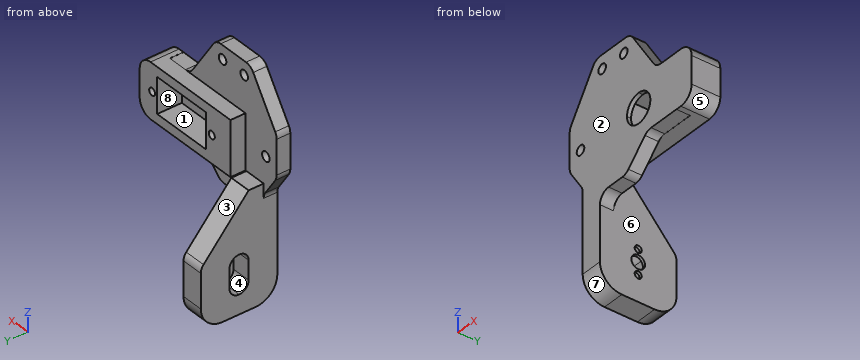
from build123d import *

# Parameters (mm, degrees)
BOSS_EXTRUDE1_DEPTH = 5
SKETCH2_R           = 1.75
SKETCH2_W           = 10.8
SKETCH2_H           = 10.8
CUT_EXTRUDE1_DEPTH  = 54.252895531
FILLET1_R           = 5.4
FILLET2_R           = 5.4
FILLET3_RADIUS      = 10
FILLET3_LENGTH      = 5
SKETCH6_W           = 35
SKETCH6_H           = 20.042215846
SKETCH6_W_2         = 23
SKETCH6_H_2         = 13
BOSS_EXTRUDE3_DEPTH = 5.5
SKETCH7_W           = 23
SKETCH7_H           = 13
CUT_EXTRUDE3_DEPTH  = 3.5
CUT_EXTRUDE4_DEPTH  = 54.302165833
SKETCH9_W           = 8
SKETCH9_H           = 28
BOSS_EXTRUDE4_DEPTH = 32
SKETCH11_R          = 2.5
SKETCH11_R_2        = 1.3
CUT_EXTRUDE5_DEPTH  = 69.854164991
FILLET6_R           = 8
BOSS_EXTRUDE5_DEPTH = 8
SKETCH13_W          = 14
SKETCH13_H          = 7
CUT_EXTRUDE6_DEPTH  = 7
FILLET7_R           = 3.5
FILLET8_R           = 3.5
CUT_EXTRUDE7_DEPTH  = 74.28896148
FILLET9_R           = 4
SKETCH15_W          = 5.3
SKETCH15_H          = 13
SKETCH15_R          = 1.4
BOSS_EXTRUDE6_DEPTH = 9
SKETCH16_W          = 7
SKETCH16_H          = 20.042215846
BOSS_EXTRUDE7_DEPTH = 10.5
SKETCH17_R          = 1.35
CUT_EXTRUDE8_DEPTH  = 9
FILLET10_R          = 5
SKETCH18_W          = 4.9
SKETCH18_H          = 13
CUT_EXTRUDE9_DEPTH  = 9


# Some blends are built 0.0001 mm under size
with BuildPart() as part:
    # Sketch1 → Boss-Extrude1 (new body)
    with BuildSketch(Plane(origin=(0, 0, 0), x_dir=(1, 0, 0), z_dir=(0, 1, 0))):
        Polygon((45, -10), (45, 10), (21, 10), (11.001510114, 19.998489886), (-4.998489886, 19.998489886), (-14.999716743, 4.996611292), (-14.999716743, -10.003388708), (-2.979747437, -28.033388708), (13.020252563, -28.033388708), (25.042481003, -10), align=None)
    extrude(amount=BOSS_EXTRUDE1_DEPTH)

    # Sketch2 → Cut-Extrude1 (cut, through all)
    with BuildSketch(Plane(origin=(0, 5, 0), x_dir=(1, 0, 0), z_dir=(0, 1, 0))):
        with Locations(Location((-9.999716743, 0, 0), (0, 0, 270))):
            Circle(SKETCH2_R)
        with Locations(Location((0.02138213, -23.033388708, 0), (0, 0, 270))):
            Circle(SKETCH2_R)
        with Locations(Location((10.02138213, -23.033388708, 0), (0, 0, 270))):
            Circle(SKETCH2_R)
        with Locations((16.9, 0)):
            Rectangle(SKETCH2_W, SKETCH2_H)
    extrude(amount=-CUT_EXTRUDE1_DEPTH, mode=Mode.SUBTRACT)

    # Fillet1
    fillet1_edges = [part.edges().sort_by_distance(p)[0] for p in [
        (11.5, 2.5, 5.4),
        (11.5, 2.5, -5.4),
    ]]
    fillet(fillet1_edges, radius=FILLET1_R - 0.0001)  # a hair under: the kernel refuses the full size

    # Fillet2
    # the kernel refuses this fillet: 5.4 mm, written as the material it adds along each edge
    with BuildSketch(Plane(origin=(22.3, 5, 5.4), x_dir=(-1, 0, 0), z_dir=(0, -1, 0)), Plane(origin=(22.3, 5, -5.4), x_dir=(0, 0, 1), z_dir=(0, -1, 0))) as fillet2_piece_1:
        with BuildLine():
            CenterArc((FILLET2_R, FILLET2_R), FILLET2_R, 180, 90)
            Line((0, FILLET2_R), (0, 0))
            Line((0, 0), (FILLET2_R, 0))
        make_face()
    extrude(amount=5)
    # the kernel refuses this fillet: 5.4 mm, written as the material it takes off along each edge

    # Fillet3: full round fillet: the end face becomes a half cylinder, R = half its width
    fillet3_face = Plane((45, 2.5, 0), x_dir=(0, 1, 0), z_dir=(1, 0, 0))  # on the end face: x along it, z out of the body
    fillet3_slab = fillet3_face.offset(-FILLET3_RADIUS / 2) * Box(FILLET3_LENGTH, 2 * FILLET3_RADIUS, FILLET3_RADIUS, mode=Mode.PRIVATE)  # the body's end, R deep
    fillet3_round = Plane((35, 2.5, 0), x_dir=(1, 0, 0), z_dir=(0, 1, 0)) * Cylinder(FILLET3_RADIUS, FILLET3_LENGTH, mode=Mode.PRIVATE)  # its axis R under the face
    add(fillet3_slab - fillet3_round, mode=Mode.SUBTRACT)

    # Sketch6 → Boss-Extrude3 (add)
    with BuildSketch(Plane(origin=(0, 5, 0), x_dir=(1, 0, 0), z_dir=(0, 1, 0))):
        with Locations((16.9, 0)):
            Rectangle(SKETCH6_W, SKETCH6_H)
        with Locations((16.9, 0)):
            Rectangle(SKETCH6_W_2, SKETCH6_H_2, mode=Mode.SUBTRACT)
    extrude(amount=BOSS_EXTRUDE3_DEPTH)

    # Sketch7 → Cut-Extrude3 (cut)
    with BuildSketch(Plane(origin=(0, 5, 0), x_dir=(1, 0, 0), z_dir=(0, 1, 0))):
        with Locations((16.9, 0)):
            Rectangle(SKETCH7_W, SKETCH7_H)
    extrude(amount=-CUT_EXTRUDE3_DEPTH, mode=Mode.SUBTRACT)

    # Sketch8 → Cut-Extrude4 (cut, through all)
    with BuildSketch(Plane(origin=(0, 5, 0), x_dir=(1, 0, 0), z_dir=(0, 1, 0))):
        with BuildLine():
            Line((34.4, 10), (34.4, -10))
            Line((34.4, -10), (35, -10))
            ThreePointArc((35, -10), (45, 0), (35, 10))
            Line((35, 10), (34.4, 10))
        make_face()
    extrude(amount=-CUT_EXTRUDE4_DEPTH, mode=Mode.SUBTRACT)

    # Sketch9 → Boss-Extrude4 (add)
    with BuildSketch(Plane(origin=(0, 0, -19.998489886), x_dir=(-1, 0, 0), z_dir=(0, 0, -1))):
        with Locations((4.998489886, 14)):
            Rectangle(SKETCH9_W, SKETCH9_H)
    extrude(amount=BOSS_EXTRUDE4_DEPTH)

    # Sketch11 → Cut-Extrude5 (cut, through all)
    with BuildSketch(Plane(origin=(-0.998489886, 0, 0), x_dir=(0, 0, -1), z_dir=(1, 0, 0))):
        with Locations((37.998489886, 14)):
            Circle(SKETCH11_R)
        with Locations((33.498489886, 14)):
            Circle(SKETCH11_R_2)
        with Locations((42.498489886, 14)):
            Circle(SKETCH11_R_2)
    extrude(amount=-CUT_EXTRUDE5_DEPTH, mode=Mode.SUBTRACT)

    # Fillet6
    fillet6_edges = [part.edges().sort_by_distance(p)[0] for p in [
        (-4.998489886, 0, -51.998489886),
        (-4.998489886, 28, -51.998489886),
    ]]
    fillet(fillet6_edges, radius=FILLET6_R)

    # Sketch12 → Boss-Extrude5 (add)
    with BuildSketch(Plane.ZY.offset(8.998489886)):
        Polygon((-10.021107923, 10.5), (-19.998489886, 28), (-19.998489886, 0), (-10, 0), align=None)
    extrude(amount=-BOSS_EXTRUDE5_DEPTH)

    # Sketch13 → Cut-Extrude6 (cut)
    with BuildSketch(Plane.ZY.offset(8.998489886)):
        with Locations((-37.998489886, 14)):
            Rectangle(SKETCH13_W, SKETCH13_H)
    extrude(amount=-CUT_EXTRUDE6_DEPTH, mode=Mode.SUBTRACT)

    # Fillet7
    fillet7_edges = [part.edges().sort_by_distance(p)[0] for p in [
        (-5.498489886, 10.5, -44.998489886),
        (-5.498489886, 17.5, -44.998489886),
    ]]
    fillet(fillet7_edges, radius=FILLET7_R - 0.0001)  # a hair under: the kernel refuses the full size

    # Fillet8
    fillet8_edges = [part.edges().sort_by_distance(p)[0] for p in [
        (-5.498489886, 17.5, -30.998489886),
        (-5.498489886, 10.5, -30.998489886),
    ]]
    fillet(fillet8_edges, radius=FILLET8_R - 0.0001)  # a hair under: the kernel refuses the full size

    # Sketch14 → Cut-Extrude7 (cut, through all)
    with BuildSketch(Plane.ZY.offset(8.998489886)):
        Polygon((-10.021107923, 10.5), (-29.998489886, 28), (-19.998489886, 28), align=None)
    extrude(amount=-CUT_EXTRUDE7_DEPTH, mode=Mode.SUBTRACT)

    # Fillet9
    # the kernel refuses this fillet: 4 mm, written as the material it adds along each edge
    with BuildSketch(Plane(origin=(-0.998489886, 5, -19.998489886), x_dir=(1, 0, 0), z_dir=(0, -1, 0))) as fillet9_piece_1:
        with BuildLine():
            CenterArc((FILLET9_R, -FILLET9_R), FILLET9_R, 90, 90)
            Line((0, -FILLET9_R), (0, 0))
            Line((0, 0), (FILLET9_R, 0))
        make_face()
    extrude(amount=5)
    with BuildSketch(Plane(origin=(25.042481003, 0, 10), x_dir=(-0.5546992156114033, 0, 0.8320509480795595), z_dir=(0, 1, 0))) as fillet9_piece_2:
        with BuildLine():
            CenterArc((FILLET9_R * 0.535184516545, FILLET9_R), FILLET9_R, 213.69, 56.31)
            Line((-FILLET9_R * 0.296866431535, FILLET9_R * 0.445300784389), (0, 0))
            Line((0, 0), (FILLET9_R * 0.535184516545, 0))
        make_face()
    extrude(amount=5)
    with BuildSketch(Plane(origin=(21, 0, -10), x_dir=(1, 0, 0), z_dir=(0, 1, 0))) as fillet9_piece_3:
        with BuildLine():
            CenterArc((FILLET9_R * 0.414213562373, FILLET9_R), FILLET9_R, 225, 45)
            Line((-FILLET9_R * 0.292893218813, FILLET9_R * 0.292893218813), (0, 0))
            Line((0, 0), (FILLET9_R * 0.414213562373, 0))
        make_face()
    extrude(amount=5)
    with BuildSketch(Plane(origin=(-8.998489886, 5, -13.998474565), x_dir=(0, 0, -1), z_dir=(0, -1, 0))) as fillet9_piece_4:
        with BuildLine():
            CenterArc((FILLET9_R * 0.302774994436, -FILLET9_R), FILLET9_R, 90, 33.69)
            Line((-FILLET9_R * 0.251924221175, -FILLET9_R * 0.16794905192), (0, 0))
            Line((0, 0), (FILLET9_R * 0.302774994436, 0))
        make_face()
    extrude(amount=5)
    # the kernel refuses this fillet: 4 mm, written as the material it takes off along each edge
    with BuildSketch(Plane(origin=(13.020252563, -5.351845165, 28.033388708), x_dir=(0.5546992156114035, 0, -0.8320509480795594), z_dir=(0, 1, 0)), Plane(origin=(-2.979747437, -5.351845165, 28.033388708), x_dir=(1, 0, 0), z_dir=(0, 1, 0))) as fillet9_2_piece_1:
        with BuildLine():
            CenterArc((FILLET9_R * 0.535184516545, FILLET9_R), FILLET9_R, 213.69, 56.31)
            Line((-FILLET9_R * 0.296866431535, FILLET9_R * 0.445300784389), (0, 0))
            Line((0, 0), (FILLET9_R * 0.535184516545, 0))
        make_face()
    extrude(amount=15.703690331, mode=Mode.SUBTRACT)
    with BuildSketch(Plane(origin=(-14.999716743, -3.027749944, 10.003388708), x_dir=(0.5546992156114036, 0, 0.8320509480795593), z_dir=(0, 1, 0)), Plane(origin=(-14.999716743, -3.027749944, -4.996611292), x_dir=(0, 0, 1), z_dir=(0, 1, 0))) as fillet9_2_piece_2:
        with BuildLine():
            CenterArc((FILLET9_R * 0.302774994436, FILLET9_R), FILLET9_R, 236.31, 33.69)
            Line((-FILLET9_R * 0.251924221175, FILLET9_R * 0.16794905192), (0, 0))
            Line((0, 0), (FILLET9_R * 0.302774994436, 0))
        make_face()
    extrude(amount=11.055499889, mode=Mode.SUBTRACT)
    with BuildSketch(Plane(origin=(11.001510114, -4.142135624, -19.998489886), x_dir=(-1, 0, 0), z_dir=(0, 1, 0))) as fillet9_2_piece_3:
        with BuildLine():
            CenterArc((FILLET9_R * 0.414213562373, FILLET9_R), FILLET9_R, 225, 45)
            Line((-FILLET9_R * 0.292893218813, FILLET9_R * 0.292893218813), (0, 0))
            Line((0, 0), (FILLET9_R * 0.414213562373, 0))
        make_face()
    extrude(amount=13.284271247, mode=Mode.SUBTRACT)
    with BuildSketch(Plane(origin=(-12.759041279, 28, -29.998489886), x_dir=(0, -0.658926553885557, 0.7522072829908683), z_dir=(1, 0, 0))) as fillet9_2_piece_4:
        with BuildLine():
            CenterArc((FILLET9_R * 0.376055139299, FILLET9_R), FILLET9_R, 228.781943012, 41.218056988)
            Line((-FILLET9_R * 0.282871414587, FILLET9_R * 0.247792717009), (0, 0))
            Line((0, 0), (FILLET9_R * 0.376055139299, 0))
        make_face()
    extrude(amount=15.521102786, mode=Mode.SUBTRACT)

    # Sketch15 → Boss-Extrude6 (add)
    with BuildSketch(Plane(origin=(0, 1.5, 0), x_dir=(1, 0, 0), z_dir=(0, 1, 0))):
        with Locations((8.05, 0)):
            Rectangle(SKETCH15_W, SKETCH15_H)
        with Locations(Location((8.05, 0, 0), (0, 0, 90))):
            Circle(SKETCH15_R, mode=Mode.SUBTRACT)
    extrude(amount=BOSS_EXTRUDE6_DEPTH)

    # Sketch16 → Boss-Extrude7 (add)
    with BuildSketch(Plane(origin=(0, 10.5, 0), x_dir=(1, 0, 0), z_dir=(0, 1, 0))):
        with Locations((37.9, 0)):
            Rectangle(SKETCH16_W, SKETCH16_H)
    extrude(amount=-BOSS_EXTRUDE7_DEPTH)

    # Sketch17 → Cut-Extrude8 (cut)
    with BuildSketch(Plane(origin=(0, 10.5, 0), x_dir=(1, 0, 0), z_dir=(0, 1, 0))):
        with Locations(Location((35.65, 0, 0), (0, 0, 270))):
            Circle(SKETCH17_R)
    extrude(amount=-CUT_EXTRUDE8_DEPTH, mode=Mode.SUBTRACT)

    # Fillet10
    fillet10_edges = [part.edges().sort_by_distance(p)[0] for p in [
        (41.4, 5.25, -10.021107923),
        (41.4, 5.25, 10.021107923),
    ]]
    fillet(fillet10_edges, radius=FILLET10_R)

    # Sketch18 → Cut-Extrude9 (cut)
    with BuildSketch(Plane(origin=(0, 10.5, 0), x_dir=(1, 0, 0), z_dir=(0, 1, 0))):
        with Locations((30.85, 0)):
            Rectangle(SKETCH18_W, SKETCH18_H)
    extrude(amount=-CUT_EXTRUDE9_DEPTH, mode=Mode.SUBTRACT)


solid = part.part
Could you check a few things on this model? Use its own coordinates, in mm. Face numbers are marked on the shaded views. A direction names the side the tool comes from. Coordinates: 2 decimals unless noted, no trailing zeros. Order: outer loops, then holes, each group sorted by start corner. A loop starts at its lowest first (then second) coordinate and runs counter-clockwise, first axis right, second up.
Q1. Suppose I cut it at D-D on z = -9. Please give me the cut outline in (x, y), and give its area (3 significant figures).
Q2. Which directions (+Z, -Z, +X, -X, +Y, -Y) give clear straight access to the entire face, cutting with the end or side of a thin tool? Please do the marked faces 4, 5, 6, 7 and 8.
Q3. Thinking about a two-plate mould opening in Z: for the marked faces 1, 2 and 3, which applies, released by +Z, released by -Z, zero draft, split by the parting line, or undercut?
Q4. Will these pins go through, and if not, where does the flat tip stop? pin 1 (3 mm diameter, centred on y = 14, z = -33.5, fed in from +X); pin 2 (2 mm diameter, centred on x = -10, z = 0, fed in from -Y); pin 3 (5.5 mm diameter, centred on x = 10.02, z = 23.03, fed in from +Y); pin 4 (10 mm diameter, centred on x = 22.5, y = 6.5, fed in from +Z).
Q5. Suppose I cut it at B-B on y = 9.25. Please give me the cut outline in (x, z), and give its area (3 significant figures).
Q6. Please list where these lines run through material, in increasing order: L1, parallel to X at y = 4.75, z = 0; L2, parallel to X at y = 1.35, z = 0; L3, parallel to Z at x = 18, y = 9.5.
Answer:
1. outline: (-12.33, 0) - (39.43, 0) - (39.43, 10.5) - (-0.6, 10.5) - (-0.6, 5) - (-12.33, 5) - close
1. area: 479 mm2
2. face 4: -X
2. face 5: -Z, +X, +Y, -Y
2. face 6: -Z, +X, +Y
2. face 7: -Z, +X, -X, -Y
2. face 8: +Y
3. face 1: undercut
3. face 2: zero draft
3. face 3: released by +Z
4. pin 1: stops at x = -1
4. pin 2: passes through
4. pin 3: stops at y = 5
4. pin 4: stops at z = 20.97
5. outline: (-9, -52) - (-1, -52) - (-1, -10.02) - (-9, -10.02) - close; (-0.6, -10.02) - (36.4, -10.02) arc R5 ccw to (41.4, -5.02) - (41.4, 5.02) arc R5 ccw to (36.4, 10.02) - (-0.6, 10.02) - close; hole circle Ø2.8 at (8.05, 0); hole (10.7, -6.5) - (33.3, -6.5) - (33.3, 6.5) - (10.7, 6.5) - close; hole circle Ø2.7 at (35.65, 0)
5. area: 861 mm2
6. L1: x = -15 to -11.75, -8.25 to 6.65, 9.45 to 10.7, 33.3 to 34.3, 37 to 41.4
6. L2: x = -15 to -11.75, -8.25 to 11.5, 22.3 to 41.4
6. L3: z = -10.02 to -6.5, 6.5 to 10.02
